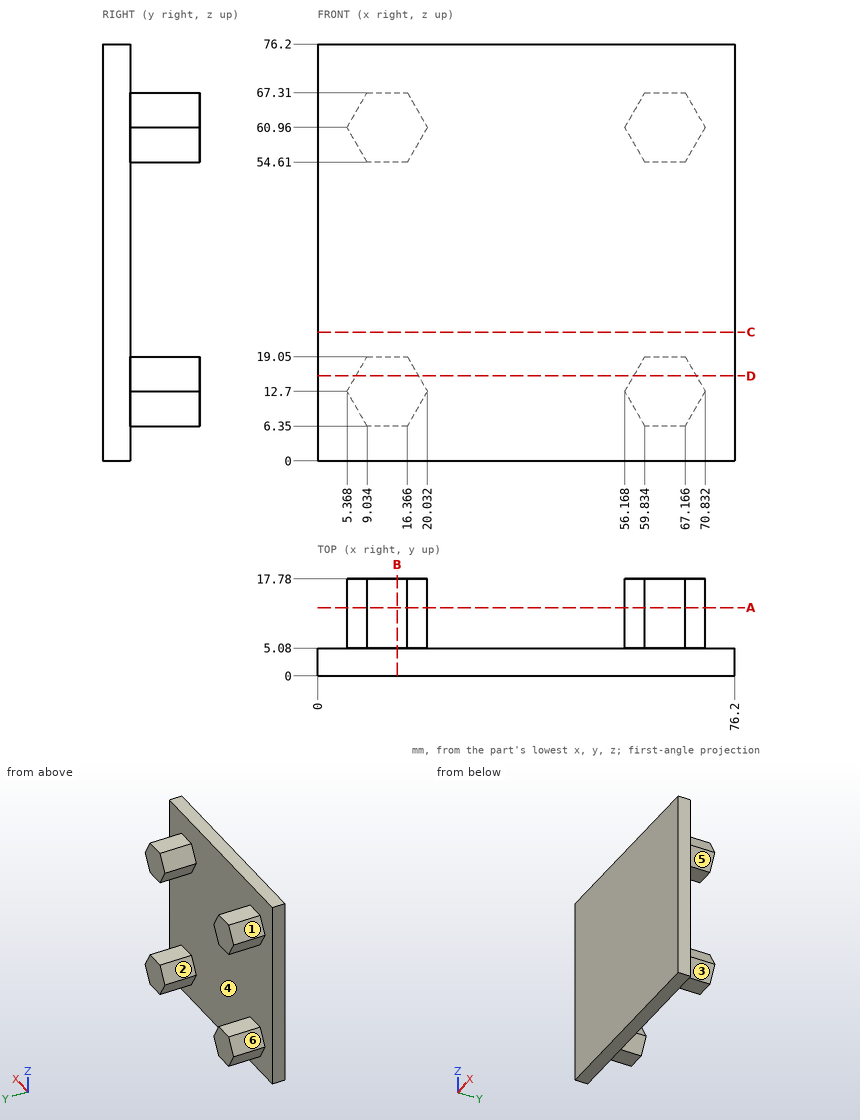
Answer from the drawing. Dimensions are ordinates in mm from the lowest x, y and z of the part. A direction names the side the tool comes from. Round coordinates to 2 decimals unless told otherwise and drop trailing zeros. Loops run counter-clockwise (first coordinate to the right, second up) from the corner with the lowest first, then second, coordinate; pieces in that order, holes last.
(1) The part is cut by section B-B, the plane x = 14.5. Give the vertices of the cut face in (y, z), and give its area (3 significant figures).
Computed values:
outline: (0, 0) - (5.08, 0) - (5.08, 6.35) - (17.78, 6.35) - (17.78, 19.05) - (5.08, 19.05) - (5.08, 54.61) - (17.78, 54.61) - (17.78, 67.31) - (5.08, 67.31) - (5.08, 76.2) - (0, 76.2) - close
area: 710 mm2
(2) The part is cut by section D-D, the plane z = 15.5. Give the vertices of the cut face in (x, y).
Computed values:
outline: (0, 0) - (76.2, 0) - (76.2, 5.08) - (69.22, 5.08) - (69.22, 17.78) - (57.78, 17.78) - (57.78, 5.08) - (18.42, 5.08) - (18.42, 17.78) - (6.98, 17.78) - (6.98, 5.08) - (0, 5.08) - close
(3) The part is cut by section A-A, the plane y = 12.5. Give the vertices of the cut face in (x, z).
Computed values:
outline: (5.37, 12.7) - (9.03, 6.35) - (16.37, 6.35) - (20.03, 12.7) - (16.37, 19.05) - (9.03, 19.05) - close; (5.37, 60.96) - (9.03, 54.61) - (16.37, 54.61) - (20.03, 60.96) - (16.37, 67.31) - (9.03, 67.31) - close; (56.17, 12.7) - (59.83, 6.35) - (67.17, 6.35) - (70.83, 12.7) - (67.17, 19.05) - (59.83, 19.05) - close; (56.17, 60.96) - (59.83, 54.61) - (67.17, 54.61) - (70.83, 60.96) - (67.17, 67.31) - (59.83, 67.31) - close
(4) Find the intervals of material crossed by L1, parallel to Z at x = 62, y = 7; L2, parallel to Y at x = 46, z = 67; L3, parallel to Z at x = 18, y = 12.75, in increasing order.
Computed values:
L1: z = 6.35 to 19.05, 54.61 to 67.31
L2: y = 0 to 5.08
L3: z = 9.18 to 16.22, 57.44 to 64.48
(5) The part is cut by section C-C, the plane z = 23.5. Give the vertices of the cut face in (x, y), and give its area (3 significant figures).
Computed values:
outline: (0, 0) - (76.2, 0) - (76.2, 5.08) - (0, 5.08) - close
area: 387 mm2
(6) The mould has two halves that part along Z. Classify the marked faces 1, 2 and 3: pulls with the +Z half, pulls with the -Z half, needs draft (parallel to the pull), parting line crosses it, or undercut.
Computed values:
face 1: pulls with the +Z half
face 2: undercut
face 3: pulls with the -Z half
(7) Each of these flat-tipped pins is pushed along its axis until it touches: P1, Ø2, axis at x = 47.5, z = 47, coming from the +Y side; P2, Ø6, axis at x = 62, y = 13, coming from the -Z side; P3, Ø2, axis at x = 11.5, y = 11.5, coming from the +Z side. Where does it stop, or does it pass through?
Computed values:
P1: stops at y = 5.08
P2: stops at z = 6.35
P3: stops at z = 67.31
(8) For the marked faces 4, 5 and 6, determine the directions among +Z, -Z, +X, -X, +Y, -Y from which every point of the face is accessible in a straight line to the end or side of a thin tool.
Computed values:
face 4: +Y
face 5: +X, +Y
face 6: -X, +Y
